Part model, mm, in its own coordinate system. Coordinates: 2 decimals unless noted, no trailing zeros. Loops run counter-clockwise (first coordinate to the right, second up) from the corner with the lowest first, then second, coordinate; pieces in that order, holes last. Notation, with made-up numbers: M 69.5,-2.75 L 111.5,-2.75 A26 cw 111.5,33.25 Z; hole C -34.75,29.5 d8. An arc over 180 degrees is marked long. Use a Markdown table: item, result. Add a question column.
1) Wall check: probe 1 along X at (y, z) = (-7.25, 0); probe 2 along X at (y, z) = (1.5, 0); probe 3 along Z at (x, y) = (-13, 1.75). Give the ranges that are in metal, low to high. Write a range as from..to.
2) Band-saw the part on D-D (x = 10.5). List the corners of the cut face in (y, z), plus the area to 3 significant figures.
3) Band-saw the part on B-B (y = -2.5). List the corners of the cut face in (x, z), plus the area to 3 significant figures.
4) Pin check, flat tips, straight feed: pin 1 Ø1 at (y, z) = (0.5, -12.5) entering from +X; pin 2 Ø1 at (x, y) = (-28.5, 1) entering from +Z; pin 3 Ø4 at (y, z) = (0.5, -35.5) entering from -X. Stop position of each tip, or through.
5) Band-saw the part on A-A (x = 45.7). List the corners of the cut face in (y, z).
6) Band-saw the part on C-C (z = -44). List the corners of the cut face in (x, y), plus the area to 3 significant figures.
from build123d import *

# Parameters (mm, degrees)
SKETCH1_W           = 36.4
SKETCH1_H           = 33
BOSS_EXTRUDE1_DEPTH = 2
SKETCH2_W           = 5
SKETCH2_H           = 4
BOSS_EXTRUDE2_DEPTH = 8
SKETCH4_R           = 1
CUT_EXTRUDE2_DEPTH  = 27.162759793
CUT_EXTRUDE1_DEPTH  = 8.5
SKETCH5_W           = 2.5
SKETCH5_H           = 2
BOSS_EXTRUDE3_DEPTH = 30
SKETCH6_W           = 2.5
SKETCH6_H           = 2
BOSS_EXTRUDE4_DEPTH = 30
SKETCH11_R          = 1.5
CUT_EXTRUDE3_DEPTH  = 52.918108594
SKETCH10_R          = 1.5
BOSS_EXTRUDE5_DEPTH = 2


with BuildPart() as part:
    # Sketch1 → Boss-Extrude1 (new body)
    with BuildSketch(Plane(origin=(0, 0, 0), x_dir=(1, 0, 0), z_dir=(0, 1, 0))):
        Rectangle(SKETCH1_W, SKETCH1_H)
        Polygon((3.667695956, -4), (15.249514138, -14.5), (0, -12.5), (-15.249514138, -14.5), (-3.667695956, -4), align=None, mode=Mode.SUBTRACT)
        Polygon((-4.412121212, -3.325108971), (-16.2, -14.011922158), (-16.2, 14.011922158), (-4.412121212, 3.325108971), align=None, mode=Mode.SUBTRACT)
        Polygon((-3.667695956, 4), (-15.249514138, 14.5), (0, 12.5), (15.249514138, 14.5), (3.667695956, 4), align=None, mode=Mode.SUBTRACT)
        Polygon((4.412121212, 3.325108971), (16.2, 14.011922158), (16.2, -14.011922158), (4.412121212, -3.325108971), align=None, mode=Mode.SUBTRACT)
    extrude(amount=BOSS_EXTRUDE1_DEPTH)

    # Sketch2 → Boss-Extrude2 (add)
    with BuildSketch(Plane.XZ):
        with Locations((15.7, 0)):
            Rectangle(SKETCH2_W, SKETCH2_H)
        with Locations((-15.7, 0)):
            Rectangle(SKETCH2_W, SKETCH2_H)
    extrude(amount=BOSS_EXTRUDE2_DEPTH)

    # Sketch4 → Cut-Extrude2 (cut, through all)
    with BuildSketch(Plane(origin=(0, 1, 0), x_dir=(1, 0, 0), z_dir=(0, 1, 0))):
        with Locations(Location((15, 0, 0), (0, 0, 270))):
            Circle(SKETCH4_R)
        with Locations(Location((-15, 0, 0), (0, 0, 270))):
            Circle(SKETCH4_R)
    extrude(amount=-CUT_EXTRUDE2_DEPTH, mode=Mode.SUBTRACT)

    # Sketch3 → Cut-Extrude1 (cut)
    with BuildSketch(Plane(origin=(0, 2, 0), x_dir=(1, 0, 0), z_dir=(0, 1, 0))):
        with BuildLine():
            Line((15, 4.124318125), (15, 4.257967602))
            Line((15, 4.257967602), (10.3221916, 4.257967602))
            Line((10.3221916, 4.257967602), (10.3221916, -5.239749404))
            Line((10.3221916, -5.239749404), (15, -5.239749404))
            Line((15, -5.239749404), (15, -4.124318125))
            ThreePointArc((15, -4.124318125), (15.326601634, -2.763090306), (16.235294118, -1.69824864))
            ThreePointArc((16.235294118, -1.69824864), (17.1, 0), (16.235294118, 1.69824864))
            ThreePointArc((16.235294118, 1.69824864), (15.326601634, 2.763090306), (15, 4.124318125))
        make_face()
        with BuildLine():
            Line((-10.3221916, -5.239749404), (-15, -5.239749404))
            Line((-15, -5.239749404), (-15, -4.124318125))
            ThreePointArc((-15, -4.124318125), (-15.326601634, -2.763090306), (-16.235294118, -1.69824864))
            ThreePointArc((-16.235294118, -1.69824864), (-17.1, 0), (-16.235294118, 1.69824864))
            ThreePointArc((-16.235294118, 1.69824864), (-15.326601634, 2.763090306), (-15, 4.124318125))
            Line((-15, 4.124318125), (-15, 4.257967602))
            Line((-15, 4.257967602), (-10.3221916, 4.257967602))
            Line((-10.3221916, 4.257967602), (-10.3221916, -5.239749404))
        make_face()
    extrude(amount=-CUT_EXTRUDE1_DEPTH, mode=Mode.SUBTRACT)

    # Sketch5 → Boss-Extrude3 (add)
    with BuildSketch(Plane.ZY.offset(18.2)):
        with Locations((1.25, 1)):
            Rectangle(SKETCH5_W, SKETCH5_H)
        with Locations((-1.25, 1)):
            Rectangle(SKETCH5_W, SKETCH5_H)
    extrude(amount=BOSS_EXTRUDE3_DEPTH)

    # Sketch6 → Boss-Extrude4 (add)
    with BuildSketch(Plane(origin=(18.2, 0, 0), x_dir=(0, 0, -1), z_dir=(1, 0, 0))):
        with Locations((-1.25, 1)):
            Rectangle(SKETCH6_W, SKETCH6_H)
        with Locations((1.25, 1)):
            Rectangle(SKETCH6_W, SKETCH6_H)
    extrude(amount=BOSS_EXTRUDE4_DEPTH)

    # Sketch11 → Cut-Extrude3 (cut, through all)
    with BuildSketch(Plane(origin=(0, 2, 0), x_dir=(1, 0, 0), z_dir=(0, 1, 0))):
        with Locations(Location((-45.7, 0, 0), (0, 0, 270))):
            Circle(SKETCH11_R)
        with Locations(Location((45.7, 0, 0), (0, 0, 270))):
            Circle(SKETCH11_R)
    extrude(amount=-CUT_EXTRUDE3_DEPTH, mode=Mode.SUBTRACT)

    # Sketch10 → Boss-Extrude5 (add)
    # profile 1 of 2: a face of its own
    with BuildSketch(Plane(origin=(0, 2, 0), x_dir=(1, 0, 0), z_dir=(0, 1, 0))):
        Polygon((0, -16.5), (-5.02079011, -16.5), (-2.27177232, -46.613981094), (2.707523657, -46.15943564), align=None)
        with Locations(Location((0, -44, 0), (0, 0, 270))):
            Circle(SKETCH10_R, mode=Mode.SUBTRACT)
    # profile 2 of 2: a face of its own
    with BuildSketch(Plane(origin=(0, 2, 0), x_dir=(1, 0, 0), z_dir=(0, 1, 0))):
        Polygon((0, 16.5), (5.02079011, 16.5), (2.27177232, 46.613981094), (-2.707523657, 46.15943564), align=None)
        with Locations(Location((0, 44, 0), (0, 0, 270))):
            Circle(SKETCH10_R, mode=Mode.SUBTRACT)
    extrude(amount=-BOSS_EXTRUDE5_DEPTH)


solid = part.part
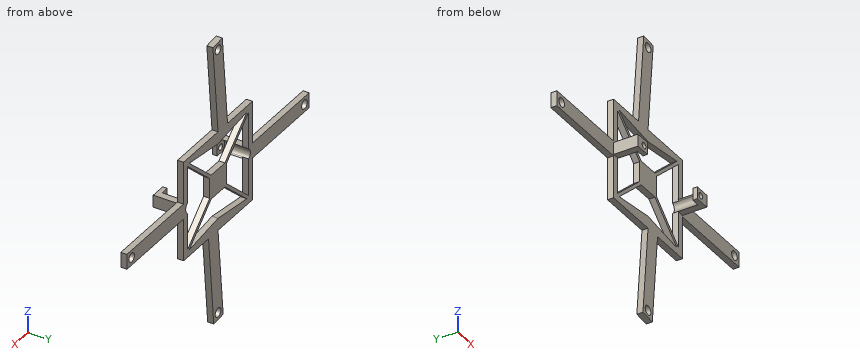
Entries:
| question | item | result |
|---|---|---|
| 1 | probe 1 | -18.2..-16, -14..-13.2, 13.2..14, 16..18.2 |
| 1 | probe 2 | -48.2..-47.2, -44.2..-17.1, -4.41..4.41, 17.1..44.2, 47.2..48.2 |
| 1 | probe 3 | -16.5..-14.2, -12.46..-11.11, 11.11..12.46, 14.2..16.5 |
| 2 | outline | M 0,-16.5 L 2,-16.5 L 2,-13.88 L 0,-13.88 Z; M 0,-10.19 L 2,-10.19 L 2,-8.84 L 0,-8.84 Z; M 0,8.84 L 2,8.84 L 2,10.19 L 0,10.19 Z; M 0,13.88 L 2,13.88 L 2,16.5 L 0,16.5 Z |
| 2 | area | 15.9 mm2 |
| 3 | outline | M -18.2,-2 L -15.88,-2 A3 ccw -16.24,-1.7 A2.1 cw -16.24,1.7 A3 ccw -15.88,2 L -18.2,2 Z; M 15.88,-2 L 18.2,-2 L 18.2,2 L 15.88,2 A3 ccw 16.24,1.7 A2.1 cw 16.24,-1.7 A3 ccw Z |
| 3 | area | 11.8 mm2 |
| 4 | pin 1 | x = 18.2 |
| 4 | pin 2 | z = 2.5 |
| 4 | pin 3 | x = -1.92 |
| 5 | outline | M 0,-2.5 L 2,-2.5 L 2,-1.5 L 0,-1.5 Z; M 0,1.5 L 2,1.5 L 2,2.5 L 0,2.5 Z |
| 6 | outline | M -2.51,0 L -1.5,0 L -1.5,2 L -2.51,2 Z; M 1.5,0 L 2.51,0 L 2.51,2 L 1.5,2 Z |
| 6 | area | 4.04 mm2 |
